```python
from build123d import *

# Parameters (mm, degrees)
SKETCH1_R           = 2.5
BOSS_EXTRUDE1_DEPTH = 5
SKETCH2_R           = 2.5
BOSS_EXTRUDE2_DEPTH = 10


with BuildPart() as part:
    # Sketch1 → Boss-Extrude1 (new body)
    with BuildSketch(Plane(origin=(0, 0, 0), x_dir=(1, 0, 0), z_dir=(0, 1, 0))):
        with BuildLine():
            Line((8.660254038, 5), (20, 5))
            ThreePointArc((20, 5), (25, 0), (20, -5))
            Line((20, -5), (8.660254038, -5))
            ThreePointArc((8.660254038, -5), (-10, 0), (8.660254038, 5))
        make_face()
        Circle(SKETCH1_R, mode=Mode.SUBTRACT)
    extrude(amount=BOSS_EXTRUDE1_DEPTH)

    # Sketch2 → Boss-Extrude2 (add)
    with BuildSketch(Plane(origin=(0, 5, 0), x_dir=(1, 0, 0), z_dir=(0, 1, 0))):
        with Locations((20, 0)):
            Circle(SKETCH2_R)
    extrude(amount=BOSS_EXTRUDE2_DEPTH)


solid = part.part
```
Here's how the part is built. I have some questions about the finished solid (model axes, mm). A direction names the side the tool comes from. Give positions to 0.01 mm unless a question says otherwise; leave off trailing zeros. Order: outer loops, then holes, each group sorted by start corner. A loop starts at its lowest first (then second) coordinate and runs counter-clockwise, first axis right, second up. Notation, with made-up numbers: (43.5, -16) - (51.5, -16) arc R8 ccw to (51.5, -11) - close; hole circle Ø7 at (84.25, 67). An arc over 180 degrees is marked (long way). Answer as a JSON object with one key per item and string values. Group by question number.
Item 1: Which directions (+Z, -Z, +X, -X, +Y, -Y) give clear straight access to the entire face, cutting with the end or side of a thin tool? Please do faces 5 (the flat face through (14, 2, 5)), 6 (the flat face through (14, 2, -5)), 7 (the flat face through (8, 0, 0)).
Item 2: If we section it at C-C on y = 2.5: Please give me the cut outline in (x, z), and give its area (3 significant figures).
Item 3: For P1, Ø4.5, axis at x = 0, z = 0, coming from the +Y side; P2, Ø6, axis at x = 1, z = 0.5, coming from the +Y side; P3, Ø3, axis at x = 3.5, y = 5, coming from the -Z side; P4, Ø4, axis at x = 11.5, y = 2, coming from the +Z side, each with a flat end and sliding along its axis, tell me the tip position at first contact or that it passes through.
Item 4: If we section it at D-D on x = 21: Please give me the cut outline in (y, z), and give its area (3 significant figures).
Item 5: Please list where these lines run through material, in increasing order: probe 1 along X at (y, z) = (2.5, 0); probe 2 along Y at (x, z) = (-1, -5); probe 3 along X at (y, z) = (2.75, -1.25).
Item 6: If we mould it in two halves opening along X, with no side actions, what happens to faces 1 (the cylindrical face through (25, 2, 0)), 2 (the cylindrical face through (17.5, 9.9, -0.1)), 3 (the cylindrical face through (-0.54, 2.46, 2.44)), 4 (the flat face through (20, 15, 0))? For each: pulls with the +X half, pulls with the -X half, needs draft (parallel to the pull), parting line crosses it, or undercut.
Item 7: If we section it at A-A on x = 0: Please give me the cut outline in (y, z).
Item 8: If we section it at B-B on z = 0: Please give me the cut outline in (x, y).
Result set:
{
 "1": {"face 5": "+Z, +X, +Y, -Y", "face 6": "-Z, +X, +Y, -Y", "face 7": "+Z, -Z, +X, -X, -Y"},
 "2": {"outline": "(8.66, -5) - (20, -5) arc R5 ccw to (20, 5) - (8.66, 5) arc R10 ccw (long way) to start; hole circle Ø5 at (0, 0)", "area": "438 mm²"},
 "3": {"P1": "through", "P2": "y = 5", "P3": "z = -9.8", "P4": "z = 5"},
 "4": {"outline": "(0, -4.9) - (5, -4.9) - (5, -2.29) - (15, -2.29) - (15, 2.29) - (5, 2.29) - (5, 4.9) - (0, 4.9) - close", "area": "94.8 mm²"},
 "5": {"probe 1": "-10 to -2.5, 2.5 to 25", "probe 2": "0 to 5", "probe 3": "-9.92 to -2.17, 2.17 to 24.84"},
 "6": {"face 1": "pulls with the +X half", "face 2": "parting line crosses it", "face 3": "undercut", "face 4": "needs draft"},
 "7": {"outline": "(0, -10) - (5, -10) - (5, -2.5) - (0, -2.5) - close; (0, 2.5) - (5, 2.5) - (5, 10) - (0, 10) - close"},
 "8": {"outline": "(-10, 0) - (-2.5, 0) - (-2.5, 5) - (-10, 5) - close; (2.5, 0) - (25, 0) - (25, 5) - (22.5, 5) - (22.5, 15) - (17.5, 15) - (17.5, 5) - (2.5, 5) - close"}
}
